```python
from build123d import *

# Parameters (mm, degrees)
SKETCH1_R           = 18.05
BOSS_EXTRUDE1_DEPTH = 3
SKETCH2_R           = 1.5
CUT_EXTRUDE1_DEPTH  = 3
CIRPATTERN1_COUNT   = 6
SKETCH3_R           = 6.05
CUT_EXTRUDE2_DEPTH  = 3
SKETCH4_W           = 39
SKETCH4_H           = 39
SKETCH4_R           = 18.05
BOSS_EXTRUDE2_DEPTH = 21
BOSS_EXTRUDE3_DEPTH = 25
SKETCH6_W           = 15
SKETCH6_H           = 10
SKETCH6_R           = 1.5
BOSS_EXTRUDE4_DEPTH = 2
SKETCH7_W           = 15
SKETCH7_H           = 10
SKETCH7_R           = 1.5
BOSS_EXTRUDE5_DEPTH = 2


with BuildPart() as part:
    # Sketch1 → Boss-Extrude1 (new body)
    with BuildSketch(Plane.XY):
        Circle(SKETCH1_R)
    extrude(amount=BOSS_EXTRUDE1_DEPTH)

    # Sketch2 → Cut-Extrude1 (cut)
    with BuildSketch(Plane.XY.offset(3)):
        with Locations((-15, 0)):
            Circle(SKETCH2_R)
    cut_extrude1 = extrude(amount=-CUT_EXTRUDE1_DEPTH, mode=Mode.SUBTRACT)

    # CirPattern1: Cut-Extrude1 ×6 about axis
    cirpattern1_axis = Axis((0, 0, 0), (0, 0, 1))
    for i in range(1, CIRPATTERN1_COUNT):
        add(cut_extrude1.rotate(cirpattern1_axis, i * 360 / CIRPATTERN1_COUNT), mode=Mode.SUBTRACT)

    # Sketch3 → Cut-Extrude2 (cut)
    with BuildSketch(Plane.XY.offset(3)):
        with Locations((0, 6)):
            Circle(SKETCH3_R)
    extrude(amount=-CUT_EXTRUDE2_DEPTH, mode=Mode.SUBTRACT)

    # Sketch4 → Boss-Extrude2 (add)
    with BuildSketch(Plane.XY.offset(3)):
        Rectangle(SKETCH4_W, SKETCH4_H)
        Circle(SKETCH4_R, mode=Mode.SUBTRACT)
    extrude(amount=-BOSS_EXTRUDE2_DEPTH)

    # Sketch5 → Boss-Extrude3 (add)
    with BuildSketch(Plane(origin=(0, 0, -18), x_dir=(-1, 0, 0), z_dir=(0, 0, -1))):
        with BuildLine():
            Line((0, 18.05), (19.5, 18.05))
            Line((19.5, 18.05), (19.5, 19.5))
            Line((19.5, 19.5), (-19.5, 19.5))
            Line((-19.5, 19.5), (-19.5, -19.5))
            Line((-19.5, -19.5), (19.5, -19.5))
            Line((19.5, -19.5), (19.5, -18.05))
            Line((19.5, -18.05), (0, -18.05))
            ThreePointArc((0, -18.05), (-18.05, 0), (0, 18.05))
        make_face()
    extrude(amount=BOSS_EXTRUDE3_DEPTH)

    # Sketch6 → Boss-Extrude4 (add)
    with BuildSketch(Plane.ZY.offset(19.5)):
        with Locations((-35.5, 24.5)):
            Rectangle(SKETCH6_W, SKETCH6_H)
        with Locations((-35.5, 24.5)):
            Circle(SKETCH6_R, mode=Mode.SUBTRACT)
        with Locations((-35.5, -24.5)):
            Rectangle(SKETCH6_W, SKETCH6_H)
        with Locations((-35.5, -24.5)):
            Circle(SKETCH6_R, mode=Mode.SUBTRACT)
    extrude(amount=-BOSS_EXTRUDE4_DEPTH)

    # Sketch7 → Boss-Extrude5 (add)
    with BuildSketch(Plane.ZY.offset(19.5)):
        with Locations((-4.5, 24.5)):
            Rectangle(SKETCH7_W, SKETCH7_H)
        with Locations((-4.5, 24.5)):
            Circle(SKETCH7_R, mode=Mode.SUBTRACT)
        with Locations((-4.5, -24.5)):
            Rectangle(SKETCH7_W, SKETCH7_H)
        with Locations((-4.5, -24.5)):
            Circle(SKETCH7_R, mode=Mode.SUBTRACT)
    extrude(amount=-BOSS_EXTRUDE5_DEPTH)


solid = part.part
```
Input: part model. Units: mm. Frame: model coordinates. A direction names the side the tool comes from. Coordinates: 2 decimals unless noted, no trailing zeros. Write each loop counter-clockwise with the first axis right and the second up, starting at its lowest first coordinate (ties: lowest second). Pieces come first, ordered by that corner, then holes.
1) Section D-D on x = -7.5. Output: boundary loops of the cut face in (y, z).
2) Pin query (flat end, axial travel): pin 1 Ø5 at (y, z) = (-24.5, -35.5) entering from +X; pin 2 Ø4 at (x, y) = (-2.5, -1.5) entering from -Z; pin 3 Ø10 at (x, z) = (-9, -36) entering from +Y. Return the tip coordinate at first contact, or that it passes through.
3) Set-up query: faces 1 (the flat face through (-18.5, 0.1, -18)), 2 (the flat face through (-17.5, 24.6, -37.3)), 3 (the flat face through (-19, 24, -28)). Return all of +Z, -Z, +X, -X, +Y, -Y with unobstructed straight access to the full face (end or side cutting, diameter ignored); none if empty.
4) Section A-A on z = -35.5. Output: boundary loops of the cut face in (x, y).
5) Mould query, pull axis X, two halves, no side actions, for faces 4 (the cylindrical face through (-18.514, 25.987, -4.695)), 5 (the cylindrical face through (16.5, -0.07, 1.52)), 6 (the flat face through (-19.5, 0, -15)). Classes: pulls with the +X half, pulls with the -X half, needs draft (parallel to the pull), parting line crosses it, or undercut.
6) Section B-B on y = -24.5. Output: boundary loops of the cut face in (x, z), and give its area (3 significant figures).
7) Material intervals for line 1 along Y through (x, z) = (7.5, 2.1); line 2 along Y through (x, z) = (-18.9, -4.5); line 3 along Y through (x, z) = (-19.05, -35.5), sorted ascending.
8) Section C-C on x = 2. Output: boundary loops of the cut face in (y, z).
Check result:
1. outline: (-19.5, -43) - (-18.05, -43) - (-18.05, -18) - (-16.42, -18) - (-16.42, 0) - (-14.49, 0) - (-14.49, 3) - (-19.5, 3) - close; (-11.49, 0) - (11.49, 0) - (11.49, 3) - (-11.49, 3) - close; (14.49, 0) - (16.42, 0) - (16.42, -18) - (18.05, -18) - (18.05, -43) - (19.5, -43) - (19.5, 3) - (14.49, 3) - close
2. pin 1: stops at x = -17.5
2. pin 2: stops at z = 0
2. pin 3: stops at y = 19.5
3. face 1: -Z, -X
3. face 2: +Z, -Z, +X, +Y
3. face 3: +X, -X, +Y
4. outline: (-19.5, -29.5) - (-17.5, -29.5) - (-17.5, -26) - (-19.5, -26) - close; (-19.5, -23) - (-17.5, -23) - (-17.5, -19.5) - (19.5, -19.5) - (19.5, 19.5) - (-17.5, 19.5) - (-17.5, 23) - (-19.5, 23) - (-19.5, 18.05) - (0, 18.05) arc R18.05 cw to (0, -18.05) - (-19.5, -18.05) - close; (-19.5, 26) - (-17.5, 26) - (-17.5, 29.5) - (-19.5, 29.5) - close
5. face 4: needs draft
5. face 5: undercut
5. face 6: pulls with the -X half
6. outline: (-19.5, -43) - (-17.5, -43) - (-17.5, -37) - (-19.5, -37) - close; (-19.5, -34) - (-17.5, -34) - (-17.5, -28) - (-19.5, -28) - close; (-19.5, -12) - (-17.5, -12) - (-17.5, -6) - (-19.5, -6) - close; (-19.5, -3) - (-17.5, -3) - (-17.5, 3) - (-19.5, 3) - close
6. area: 48.0 mm2
7. line 1: y = -19.5 to -14.49, -11.49 to 11.49, 14.49 to 19.5
7. line 2: y = -29.5 to -26, -23 to 23, 26 to 29.5
7. line 3: y = -29.5 to -26, -23 to -18.05, 18.05 to 23, 26 to 29.5
8. outline: (-19.5, -43) - (-17.94, -43) - (-17.94, 0) - (0.29, 0) - (0.29, 3) - (-19.5, 3) - close; (11.71, 0) - (17.94, 0) - (17.94, -43) - (19.5, -43) - (19.5, 3) - (11.71, 3) - close
